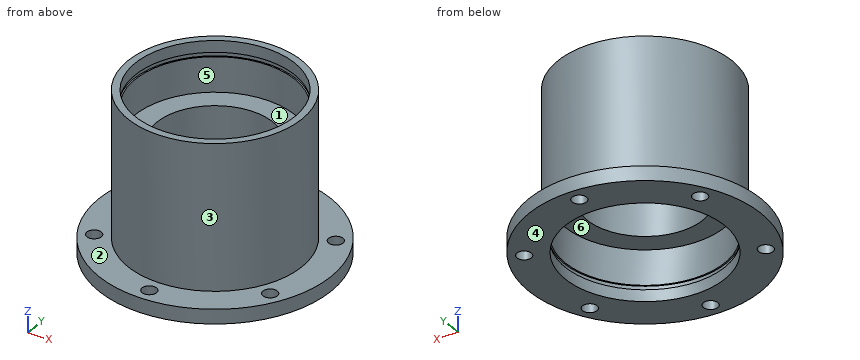
from build123d import *
from build123d.topology import SkipClean

# Parameters (mm, degrees)
SKETCH1_R                = 40
SKETCH1_R_2              = 2.5
BOSS_EXTRUDE1_DEPTH      = 5
SKETCH2_R                = 30
SKETCH2_R_2              = 27.5
BOSS_EXTRUDE2_DEPTH      = 50
SKETCH3_R                = 27.5
CUT_EXTRUDE1_DEPTH       = 50
BOSS_EXTRUDE4_DEPTH      = 10
BOSS_EXTRUDE4_DEPTH_BACK = 10
SKETCH5_R                = 27.5
SKETCH5_R_2              = 20
CUT_EXTRUDE2_START       = 12
SKETCH6_R                = 28
CUT_EXTRUDE2_DEPTH       = 1.5
CUT_EXTRUDE3_START       = 13.5
SKETCH7_R                = 28
CUT_EXTRUDE3_DEPTH       = 1.5


with BuildPart() as part:
    # Sketch1 → Boss-Extrude1 (new body)
    with BuildSketch(Plane.XY):
        Circle(SKETCH1_R)
        with Locations((0, 35)):
            Circle(SKETCH1_R_2, mode=Mode.SUBTRACT)
        with Locations((30.310889132, 17.5)):
            Circle(SKETCH1_R_2, mode=Mode.SUBTRACT)
        with Locations((30.310889132, -17.5)):
            Circle(SKETCH1_R_2, mode=Mode.SUBTRACT)
        with Locations((0, -35)):
            Circle(SKETCH1_R_2, mode=Mode.SUBTRACT)
        with Locations((-30.310889132, -17.5)):
            Circle(SKETCH1_R_2, mode=Mode.SUBTRACT)
        with Locations((-30.310889132, 17.5)):
            Circle(SKETCH1_R_2, mode=Mode.SUBTRACT)
    extrude(amount=BOSS_EXTRUDE1_DEPTH)

    # Sketch2 → Boss-Extrude2 (add)
    with BuildSketch(Plane.XY.offset(5)):
        Circle(SKETCH2_R)
        Circle(SKETCH2_R_2, mode=Mode.SUBTRACT)
    extrude(amount=BOSS_EXTRUDE2_DEPTH)

    # Sketch3 → Cut-Extrude1 (cut)
    with SkipClean():  # the faces are left unmerged after this step: merging them gives an invalid solid
        with BuildSketch(Plane(origin=(0, 0, 0), x_dir=(-1, 0, 0), z_dir=(0, 0, -1))):
            Circle(SKETCH3_R)
        extrude(amount=-CUT_EXTRUDE1_DEPTH, mode=Mode.SUBTRACT)

    # Sketch5 → Boss-Extrude4 (add, two sides: drawn at the far end of the back side and taken through both)
    with BuildSketch(Plane(origin=(0, 0, 27.5), x_dir=(-1, 0, 0), z_dir=(0, 0, -1)).offset(-BOSS_EXTRUDE4_DEPTH_BACK)):
        Circle(SKETCH5_R)
        Circle(SKETCH5_R_2, mode=Mode.SUBTRACT)
    extrude(amount=BOSS_EXTRUDE4_DEPTH + BOSS_EXTRUDE4_DEPTH_BACK)

    # Sketch6 → Cut-Extrude2 (cut)
    with BuildSketch(Plane(origin=(0, 0, 17.5), x_dir=(-1, 0, 0), z_dir=(0, 0, -1)).offset(CUT_EXTRUDE2_START)):
        with Locations(Location((0, 0, 0), (0, 0, 180))):
            Circle(SKETCH6_R)
    extrude(amount=CUT_EXTRUDE2_DEPTH, mode=Mode.SUBTRACT)

    # Sketch7 → Cut-Extrude3 (cut)
    with BuildSketch(Plane.XY.offset(37.5).offset(CUT_EXTRUDE3_START)):
        Circle(SKETCH7_R)
    extrude(amount=-CUT_EXTRUDE3_DEPTH, mode=Mode.SUBTRACT)


solid = part.part
Can you work these out from the model? Positions are in its coordinate system, mm. Face numbers are marked on the shaded views. A direction names the side the tool comes from. Coordinates: 2 decimals unless noted, no trailing zeros. Loops run counter-clockwise (first coordinate to the right, second up) from the corner with the lowest first, then second, coordinate; pieces in that order, holes last. Notation, with made-up numbers: (3, 38) - (28, 38) arc R17 ccw to (28, 63) - close; hole circle Ø2 at (41, 68.5). An arc over 180 degrees is marked (long way). Answer as a JSON object with one key per item and string values. Group by question number.
Item 1: For pin 1 (3 mm diameter, centred on y = -22, z = 18, fed in from -X); pin 2 (8 mm diameter, centred on x = 30.31, y = -17.5, fed in from +Z); pin 3 (12 mm diameter, centred on x = -26.5, z = 23, fed in from +Y); pin 4 (17 mm diameter, centred on x = -2.5, y = 4.5, fed in from +Z), each with a flat end and sliding along its axis, tell me the tip position at first contact or that it passes through.
Item 2: If we section it at C-C (z = 28): List the corners of the cut face in (x, y) for me.
Item 3: If we section it at A-A (y = -35): List the corners of the cut face in (x, z) for me.
Item 4: On a 3-axis mill with a long thin cutter (end or side, diameter ignored), from which of +Z, -Z, +X, -X, +Y, -Y can I reach the whole of each face in a straight line? I mean the marked faces 4, 5 and 6. Say none if no direction works.
Item 5: If we section it at B-B (x = 0): State how many separate pieces and enclosed holes the cut face has, plus the area to 3 significant figures.
Item 6: If I drill on L1, parallel to Y at x = 0, z = 4.4; L2, parallel to Y at x = 0, z = 2; L3, parallel to Y at x = 0, z = 53, over which ranges is the centre line in solid material (lowest first)? Write a range as from..to.
Item 7: If we mould it in two halves opening along X, with no side actions, what happens to the marked faces 1, 2 and 3? For each: released by +X, released by -X, zero draft, split by the parting line, or undercut.
Returned:
{
 "1": {"pin 1": "stops at x = -21.9", "pin 2": "stops at z = 5", "pin 3": "stops at y = 21.9", "pin 4": "passes through"},
 "2": {"outline": "circle Ø60 at (0, 0); hole circle Ø40 at (0, 0)"},
 "3": {"outline": "(-19.36, 0) - (-2.5, 0) - (-2.5, 5) - (-19.36, 5) - close; (2.5, 0) - (19.36, 0) - (19.36, 5) - (2.5, 5) - close"},
 "4": {"face 4": "-Z, +X, -X, +Y, -Y", "face 5": "+Z", "face 6": "-Z"},
 "5": {"separate pieces": "4", "enclosed holes": "0", "area": "622 mm²"},
 "6": {"L1": "y = -40..-37.5, -32.5..-28, 28..32.5, 37.5..40", "L2": "y = -40..-37.5, -32.5..-27.5, 27.5..32.5, 37.5..40", "L3": "y = -30..-27.5, 27.5..30"},
 "7": {"face 1": "undercut", "face 2": "zero draft", "face 3": "split by the parting line"}
}
